Study the drawing (mm; zero at the part's minimum x, y, z) and answer. A direction names the side the tool comes from. Give positions to 0.01 mm unless a question says otherwise; leave off trailing zeros. Write each loop counter-clockwise with the first axis right and the second up, starting at its lowest first coordinate (ties: lowest second). Pieces come first, ordered by that corner, then holes. Notation, with made-up numbers: (30.5, -23) - (88.5, -23) arc R20 ccw to (88.5, -8) - close; hole circle Ø6 at (79, 3). An arc over 180 degrees is marked (long way). Write each question's results on one line, items separated by ' | '. Start each with the question number.
Q1. Flat-ended cylindrical pins translate along their axes: pin 1 Ø6 at (x, z) = (49.5, 7.5) entering from +Y; pin 2 Ø6 at (x, z) = (32.5, 2) entering from -Y (1 decimal); pin 3 Ø1.5 at (x, z) = (26.5, 4) entering from -Y. Find the tip coordinate at first contact, or state that the pin passes through.
Q2. Section A-A (z = 1.5) is taken. Determine the outline of the cut face in (x, y).
Q3. For the marked faces 1 and 2, determine the directions among +Z, -Z, +X, -X, +Y, -Y from which every point of the face is accessible in a straight line to the end or side of a thin tool.
Q4. Find the intervals of material crossed by probe 1 along Z at (x, y) = (56, 60); probe 2 along Y at (x, z) = (36, 2.75) (1 decimal); probe 3 along X at (y, z) = (44.5, 1.5) (1 decimal), in increasing order.
Q5. Section B-B (z = 11.25) is taken. Determine the outline of the cut face in (x, y) (1 decimal).
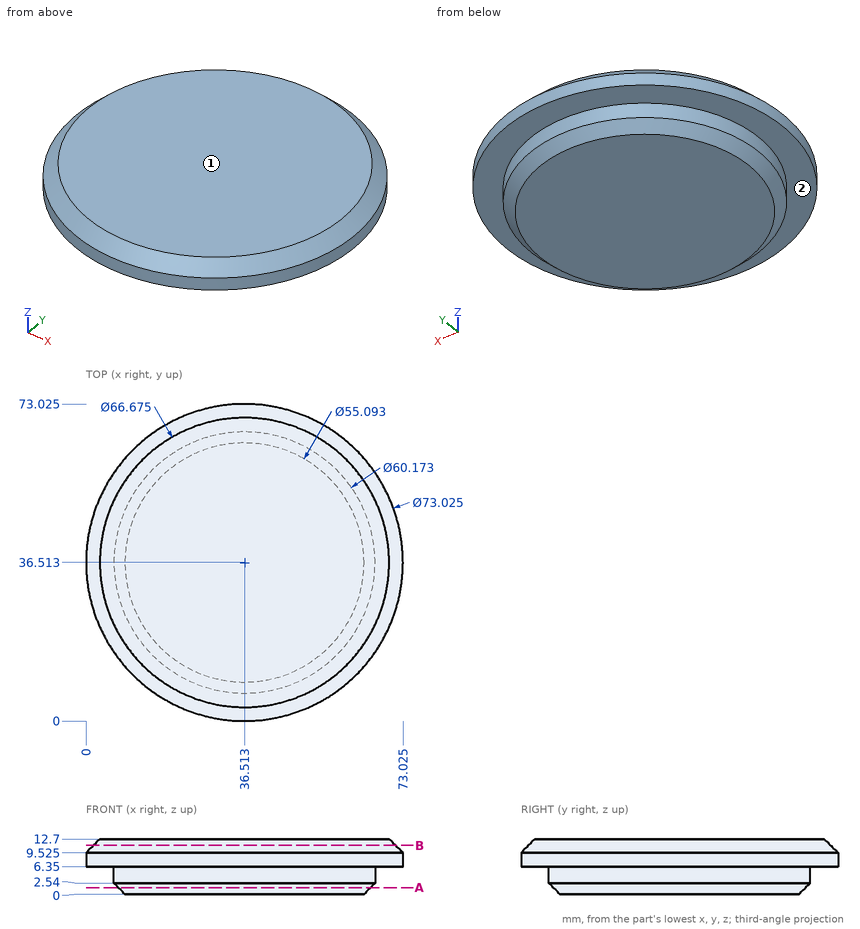
Answers below:
1) pin 1: stops at y = 71.63 | pin 2: stops at y = 6.4 | pin 3: stops at y = 7.89
2) outline: circle Ø58.09 at (36.51, 36.51)
3) face 1: +Z, +X, -X, +Y, -Y | face 2: -Z
4) probe 1: z = 6.35 to 12.7 | probe 2: y = 6.4 to 66.6 | probe 3: x = 8.6 to 64.4
5) outline: circle Ø69.6 at (36.5, 36.5)
